Part model, mm, in its own coordinate system. Face numbers are marked on the shaded views. Give positions to 0.01 mm unless a question says otherwise; leave off trailing zeros. Write each loop counter-clockwise with the first axis right and the second up, starting at its lowest first coordinate (ties: lowest second). Pieces come first, ordered by that corner, then holes. Notation, with made-up numbers: M 43,59 L 81,59 A17 cw 81,73 Z; hole C 19.5,-26.5 d11. An arc over 180 degrees is marked long. Use CSV: the item, a comma, the result in double quotes. Start each with the question number.
1. Band-saw the part on A-A, the plane x = 15.5. List the corners of the cut face in (y, z).
2. Drill centre lines: line 1 along Z through (x, y) = (3, 12.25); line 2 along Z through (x, y) = (15.5, 3.5); line 3 along Y through (x, z) = (21.1, 17.5). Where is each one in solid material? Low to high. Write a range as from..to.
3. Drop flat-ended pins along their axis: pin 1 Ø2.5 at (x, z) = (15.5, -17.5) entering from -Y; pin 2 Ø14 at (y, z) = (12.5, -17.5) entering from +X; pin 3 Ø6 at (y, z) = (17, -15) entering from -X. Give the stop position or say it passes through.
4. Band-saw the part on B-B, the plane z = -17.5. List the corners of the cut face in (x, y).
5. Band-saw the part on C-C, the plane y = 13.75. Count the separate pieces of the cut face and the enclosed holes in it, then the cut area to 3 significant figures.
6. Mould opens along Y. For the marked faces 1, 2, 3 and 4 say: pulls with the +Y half, pulls with the -Y half, needs draft (parallel to the pull), parting line crosses it, or undercut.
from build123d import *

# Parameters (mm, degrees)
SKETCH1_W                = 45
SKETCH1_H                = 102
BOSS_EXTRUDE1_DEPTH      = 25
M5_TAPPED_HOLE3_D        = 4.2
SKETCH27_R               = 6
CUT_EXTRUDE1_DEPTH       = 74
SKETCH28_R               = 10
CUT_EXTRUDE3_DEPTH       = 2
SKETCH30_R               = 10
CUT_EXTRUDE4_DEPTH       = 2
M5_TAPPED_HOLE4_D        = 4.2
M5_TAPPED_HOLE4_DEPTH    = 14
M5_TAPPED_HOLE4_TIP      = 1.2618073
M5_TAPPED_HOLE5_D        = 4.2
M5_TAPPED_HOLE5_DEPTH    = 15
M5_TAPPED_HOLE5_TIP      = 1.2618073
CUT_EXTRUDE5_DEPTH       = 1.0000001
CUT_EXTRUDE5_DEPTH_BACK  = 26.0000001
CUT_EXTRUDE12_DEPTH      = 1.0000001
CUT_EXTRUDE12_DEPTH_BACK = 26.0000001
M5_TAPPED_HOLE6_D        = 4.2
M5_TAPPED_HOLE6_DEPTH    = 15
M5_TAPPED_HOLE6_TIP      = 1.2618073


with BuildPart() as part:
    # Sketch1 → Boss-Extrude1 (new body)
    with BuildSketch(Plane(origin=(0, 0, 0), x_dir=(1, 0, 0), z_dir=(0, 1, 0))):
        Rectangle(SKETCH1_W, SKETCH1_H)
    extrude(amount=BOSS_EXTRUDE1_DEPTH)

    # M5 Tapped Hole3 (through all)
    with Locations(Plane(origin=(0, 25, 0), x_dir=(1, 0, 0), z_dir=(0, 1, 0))):
        with Locations((15.5, 17.5), (15.5, -17.5)):
            Hole(M5_TAPPED_HOLE3_D / 2)

    # Sketch27 → Cut-Extrude1 (cut)
    with BuildSketch(Plane.ZY.offset(22.5)):
        with Locations((-17.5, 12.5)):
            Circle(SKETCH27_R)
        with Locations((17.5, 12.5)):
            Circle(SKETCH27_R)
    extrude(amount=-CUT_EXTRUDE1_DEPTH, mode=Mode.SUBTRACT)

    # Sketch28 → Cut-Extrude3 (cut)
    with BuildSketch(Plane.ZY.offset(22.5)):
        with Locations((-17.5, 12.5)):
            Circle(SKETCH28_R)
        with Locations((17.5, 12.5)):
            Circle(SKETCH28_R)
    extrude(amount=-CUT_EXTRUDE3_DEPTH, mode=Mode.SUBTRACT)

    # Sketch30 → Cut-Extrude4 (cut)
    with BuildSketch(Plane(origin=(22.5, 0, 0), x_dir=(0, 0, -1), z_dir=(1, 0, 0))):
        with Locations((-17.5, 12.5)):
            Circle(SKETCH30_R)
        with Locations((17.5, 12.5)):
            Circle(SKETCH30_R)
    extrude(amount=-CUT_EXTRUDE4_DEPTH, mode=Mode.SUBTRACT)

    # M5 Tapped Hole4
    with Locations(Plane(origin=(0, 0, -51), x_dir=(-1, 0, 0), z_dir=(0, 0, -1))):
        with Locations((-18, 5), (18, 20)):
            Hole(M5_TAPPED_HOLE4_D / 2, depth=M5_TAPPED_HOLE4_DEPTH)
            with Locations((0, 0, -(M5_TAPPED_HOLE4_DEPTH + M5_TAPPED_HOLE4_TIP / 2))):  # 118° drill point
                Cone(0, M5_TAPPED_HOLE4_D / 2, M5_TAPPED_HOLE4_TIP, mode=Mode.SUBTRACT)

    # M5 Tapped Hole5
    with Locations(Plane.ZY.offset(22.5)):
        with Locations((0, 12.5)):
            Hole(M5_TAPPED_HOLE5_D / 2, depth=M5_TAPPED_HOLE5_DEPTH)
            with Locations((0, 0, -(M5_TAPPED_HOLE5_DEPTH + M5_TAPPED_HOLE5_TIP / 2))):  # 118° drill point
                Cone(0, M5_TAPPED_HOLE5_D / 2, M5_TAPPED_HOLE5_TIP, mode=Mode.SUBTRACT)

    # Sketch37 → Cut-Extrude5 (cut, two sides)
    with BuildSketch(Plane(origin=(0, 25, 0), x_dir=(1, 0, 0), z_dir=(0, 1, 0))) as cut_extrude5_sk:
        Polygon((-226.623671921, 35), (-22.5, 35), (22.5, 35), (226.623671921, 35), (226.623671921, 443.247343842), (-226.623671921, 443.247343842), align=None)
    extrude(amount=CUT_EXTRUDE5_DEPTH, mode=Mode.SUBTRACT)
    extrude(cut_extrude5_sk.sketch, amount=-CUT_EXTRUDE5_DEPTH_BACK, mode=Mode.SUBTRACT)

    # Sketch38 → Cut-Extrude12 (cut, two sides)
    with BuildSketch(Plane(origin=(0, 25, 0), x_dir=(1, 0, 0), z_dir=(0, 1, 0))) as cut_extrude12_sk:
        Polygon((-198.933169771, -35), (-22.5, -35), (22.5, -35), (198.933169771, -35), (198.933169771, -387.866339542), (-198.933169771, -387.866339542), align=None)
    extrude(amount=CUT_EXTRUDE12_DEPTH, mode=Mode.SUBTRACT)
    extrude(cut_extrude12_sk.sketch, amount=-CUT_EXTRUDE12_DEPTH_BACK, mode=Mode.SUBTRACT)

    # M5 Tapped Hole6
    with Locations(Plane.ZY.offset(22.5)):
        with Locations((-29, 5), (29, 20)):
            Hole(M5_TAPPED_HOLE6_D / 2, depth=M5_TAPPED_HOLE6_DEPTH)
            with Locations((0, 0, -(M5_TAPPED_HOLE6_DEPTH + M5_TAPPED_HOLE6_TIP / 2))):  # 118° drill point
                Cone(0, M5_TAPPED_HOLE6_D / 2, M5_TAPPED_HOLE6_TIP, mode=Mode.SUBTRACT)


solid = part.part
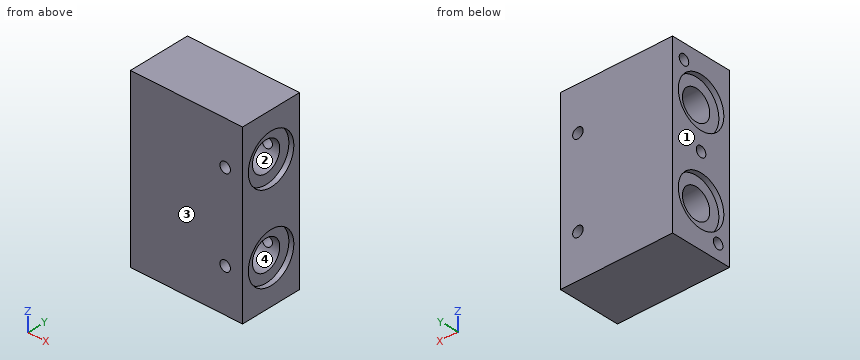
Output:
1,outline,"M 0,-35 L 25,-35 L 25,-19.6 L 18.12,-19.6 A6 cw 6.88,-19.6 L 0,-19.6 Z; M 0,-15.4 L 6.88,-15.4 A6 cw 18.12,-15.4 L 25,-15.4 L 25,15.4 L 18.12,15.4 A6 cw 6.88,15.4 L 0,15.4 Z; M 0,19.6 L 6.88,19.6 A6 cw 18.12,19.6 L 25,19.6 L 25,35 L 0,35 Z"
2,line 1,"z = -35..-23.49, -11.51..11.51, 23.49..35"
2,line 2,"z = -35..-19.6, -15.4..15.4, 19.6..35"
2,line 3,"y = 0..2.5, 22.5..25"
3,pin 1,"passes through"
3,pin 2,"stops at x = 20.5"
3,pin 3,"stops at x = -20.5"
4,outline,"M -22.5,0 L 13.4,0 L 13.4,6.5 L -20.5,6.5 L -20.5,2.5 L -22.5,2.5 Z; M -22.5,22.5 L -20.5,22.5 L -20.5,18.5 L 13.4,18.5 L 13.4,25 L -22.5,25 Z; M 17.6,0 L 22.5,0 L 22.5,2.5 L 20.5,2.5 L 20.5,6.5 L 17.6,6.5 Z; M 17.6,18.5 L 20.5,18.5 L 20.5,22.5 L 22.5,22.5 L 22.5,25 L 17.6,25 Z"
5,separate pieces,"3"
5,enclosed holes,"0"
5,area,"1,980 mm²"
6,face 1,"needs draft"
6,face 2,"undercut"
6,face 3,"pulls with the -Y half"
6,face 4,"undercut"
